Here's how the part is built. I have some questions about the finished solid (model axes, mm). A direction names the side the tool comes from. Give positions to 0.01 mm unless a question says otherwise; leave off trailing zeros. Loops run counter-clockwise (first coordinate to the right, second up) from the corner with the lowest first, then second, coordinate; pieces in that order, holes last.
Q1. Thinking about a two-plate mould opening in X: for faces 1 (the face through (39.6, 61.94, 12.68)), 2 (the face through (10, 50, 5)), 3 (the face through (20, 39, 25)), which applies, pulls with the +X half, pulls with the -X half, needs draft (parallel to the pull), parting line crosses it, or undercut?
Q2. I need wall thicknesses on probe 1 along Y at (x, z) = (10, 12); probe 2 along Y at (x, z) = (10, 16); probe 3 along Y at (x, z) = (10, 21.25). Which ranges of each line are inside material? Lowest first, please.
Q3. Suppose I cut it at B-B (x = 4). List the corners of the cut face in (y, z) for me.
Q4. I'm going to push flat-ended pins straight in: P1, Ø3, axis at x = 37.5, y = 28, coming from the +Z side; P2, Ø3, axis at x = 4, z = 16.5, coming from the -Y side; P3, Ø5, axis at x = 11.5, y = 31.5, coming from the +Z side. Where does each tip first touch, or does it pass through?
Q5. For faces 4 (the face through (30, 42, 20.1)), 5 (the face through (35, 36.14, 22)), 6 (the face through (29.25, 56, 17)), 7 (the face through (9.9, 28.8, 5)), which set-ups out of +Z, -Z, +X, -X, +Y, -Y let a thin tool reach every point of the face, with its end or its side?
Q6. Suppose I cut it at D-D (y = 41.65). List the corners of the cut face in (x, z) for me.
Q7. Suppose I cut it at A-A (y = 52.3). List the corners of the cut face in (x, z) for me, and give its area (4 significant figures).
Q8. Suppose I cut it at C-C (z = 15). List the corners of the cut face in (x, y) for me.
```python
from build123d import *

# Parameters (mm, degrees)
EXTRUDE_DEPTH     = 20
BOX003_W          = 15
BOX003_H          = 7.5
BOX003_DEPTH      = 6
CYLINDER003_R     = 2.1
CYLINDER003_DEPTH = 5
CYLINDER002_R     = 1.05
CYLINDER002_DEPTH = 7
BOX002_W          = 10
BOX002_H          = 13
BOX002_DEPTH      = 6
CYLINDER001_R     = 2
CYLINDER001_DEPTH = 5
CYLINDER_R        = 5
CYLINDER_DEPTH    = 20
BOX001_W          = 20.5
BOX001_H          = 20.5
BOX001_DEPTH      = 25
BOX004_W          = 7.5
BOX004_H          = 13
BOX004_DEPTH      = 6
BOX_W             = 40.5
BOX_H             = 62.8
BOX_DEPTH         = 25
FILLET_R          = 3


with BuildPart() as obj1:
    # Sketch → Extrude (new body)
    with BuildSketch(Plane.YZ):
        with BuildLine():
            ThreePointArc((-3.606243, 3.606246), (0, -5.1), (3.606243, 3.606246))
            Line((2.112489, 5.1), (3.606243, 3.606246))
            Line((-2.112489, 5.1), (2.112489, 5.1))
            Line((-3.606243, 3.606246), (-2.112489, 5.1))
        make_face()
    extrude(amount=EXTRUDE_DEPTH)


with BuildPart() as obj1_1:
    # Extrude placement: moved
    add(obj1.part.moved(Location((20.5, 41.65, 15))))


with BuildPart() as hueco_taladro4:
    # Box003 → Box003 (new body)
    with BuildSketch(Plane(origin=(0, 39, 14), x_dir=(1, 0, 0), z_dir=(0, 0, 1))):
        with Locations((7.5, 3.75)):
            Rectangle(BOX003_W, BOX003_H)
    extrude(amount=BOX003_DEPTH)


with BuildPart() as taladro4:
    # Cylinder003 → Cylinder003 (new body)
    with BuildSketch(Plane(origin=(10, 42.7, 20), x_dir=(1, 0, 0), z_dir=(0, 0, 1))):
        Circle(CYLINDER003_R)
    extrude(amount=CYLINDER003_DEPTH)


with BuildPart() as clone005:
    # Clone005 base: copy of taladro4
    add(taladro4.part)


with BuildPart() as clone005_1:
    # Clone005 placement: moved
    add(clone005.part.moved(Location((15.5, 13.1, 0))))


with BuildPart() as taladro_endstop:
    # Cylinder002 → Cylinder002 (new body)
    with BuildSketch(Plane(origin=(35.5, 26.14, 12), x_dir=(1, 0, 0), z_dir=(0, 0, 1))):
        Circle(CYLINDER002_R)
    extrude(amount=CYLINDER002_DEPTH)


with BuildPart() as clone004:
    # Clone004 base: copy of taladro_endstop
    add(taladro_endstop.part)


with BuildPart() as clone004_1:
    # Clone004 placement: moved
    add(clone004.part.moved(Location((0, 7, 0))))


with BuildPart() as hueco_endstop:
    # Box002 → Box002 (new body)
    with BuildSketch(Plane(origin=(30.5, 23.14, 19), x_dir=(1, 0, 0), z_dir=(0, 0, 1))):
        with Locations((5, 6.5)):
            Rectangle(BOX002_W, BOX002_H)
    extrude(amount=BOX002_DEPTH)


with BuildPart() as taladro5:
    # Cylinder001 → Cylinder001 (new body)
    with BuildSketch(Plane(origin=(30.5, 10, 0), x_dir=(1, 0, 0), z_dir=(0, 0, 1))):
        Circle(CYLINDER001_R)
    extrude(amount=CYLINDER001_DEPTH)


with BuildPart() as clone002:
    # Clone002 base: copy of taladro5
    add(taladro5.part)


with BuildPart() as clone002_1:
    # Clone002 placement: moved
    add(clone002.part.moved(Location((-20.5, 21, 0))))


with BuildPart() as clone003:
    # Clone003 base: copy of Clone002
    add(clone002_1.part)


with BuildPart() as clone003_1:
    # Clone003 placement: moved
    add(clone003.part.moved(Location((0, 21.3, 0))))


with BuildPart() as taladro10:
    # Cylinder → Cylinder (new body)
    with BuildSketch(Plane(origin=(30.5, 10, 5), x_dir=(1, 0, 0), z_dir=(0, 0, 1))):
        Circle(CYLINDER_R)
    extrude(amount=CYLINDER_DEPTH)


with BuildPart() as clone:
    # Clone base: copy of taladro10
    add(taladro10.part)


with BuildPart() as clone_1:
    # Clone placement: moved
    add(clone.part.moved(Location((-20.5, 21, 0))))


with BuildPart() as clone001:
    # Clone001 base: copy of Clone
    add(clone_1.part)


with BuildPart() as clone001_1:
    # Clone001 placement: moved
    add(clone001.part.moved(Location((0, 21.3, 0))))


with BuildPart() as obj2:
    # Box001 → Box001 (new body)
    with BuildSketch(Plane.XY):
        with Locations((10.25, 10.25)):
            Rectangle(BOX001_W, BOX001_H)
    extrude(amount=BOX001_DEPTH)


with BuildPart() as huecos:
    # Box004 → Box004 (new body)
    with BuildSketch(Plane(origin=(21.75, 49.8, 14), x_dir=(1, 0, 0), z_dir=(0, 0, 1))):
        with Locations((3.75, 6.5)):
            Rectangle(BOX004_W, BOX004_H)
    extrude(amount=BOX004_DEPTH)

    # Fusion: union hueco_taladro4, Clone005, taladro4, Clone004, taladro_endstop, hueco_endstop, Clone003, Clone002, taladro5, Clone001, Clone, taladro10, obj2
    add(hueco_taladro4.part)
    add(clone005_1.part)
    add(taladro4.part)
    add(clone004_1.part)
    add(taladro_endstop.part)
    add(hueco_endstop.part)
    add(clone003_1.part)
    add(clone002_1.part)
    add(taladro5.part)
    add(clone001_1.part)
    add(clone_1.part)
    add(taladro10.part)
    add(obj2.part)


with BuildPart() as obj3:
    # Box → Box (new body)
    with BuildSketch(Plane.XY):
        with Locations((20.25, 31.4)):
            Rectangle(BOX_W, BOX_H)
    extrude(amount=BOX_DEPTH)

    # Cut: cut huecos
    add(huecos.part, mode=Mode.SUBTRACT)

    # Cut001: cut obj1
    add(obj1_1.part, mode=Mode.SUBTRACT)

    # Fillet
    fillet_edges = [obj3.edges().sort_by_distance(p)[0] for p in [
        (0, 62.8, 12.5),
        (40.5, 62.8, 12.5),
        (40.5, 0, 12.5),
    ]]
    fillet(fillet_edges, radius=FILLET_R)


solid = obj3.part
```
Solutions:
1. face 1: pulls with the +X half
1. face 2: undercut
1. face 3: needs draft
2. probe 1: y = 20.5 to 26, 36 to 47.3, 57.3 to 62.8
2. probe 2: y = 20.5 to 26, 36 to 39, 46.5 to 47.3, 57.3 to 62.8
2. probe 3: y = 20.5 to 26, 36 to 40.6, 44.8 to 47.3, 57.3 to 62.8
3. outline: (20.5, 0) - (62.8, 0) - (62.8, 25) - (20.5, 25) - close; hole (39, 14) - (46.5, 14) - (46.5, 20) - (39, 20) - close
4. P1: stops at z = 19
4. P2: stops at y = 20.5
4. P3: stops at z = 5
5. face 4: +X
5. face 5: +Z, +X
5. face 6: +Y
5. face 7: +Z
6. outline: (0, 0) - (40.5, 0) - (40.5, 9.9) - (20.5, 9.9) - (20.5, 20.1) - (40.5, 20.1) - (40.5, 25) - (11.82, 25) - (11.82, 20) - (15, 20) - (15, 14) - (0, 14) - close; (0, 20) - (8.18, 20) - (8.18, 25) - (0, 25) - close
7. outline: (0, 0) - (8, 0) - (8, 5) - (5, 5) - (5, 25) - (0, 25) - close; (12, 0) - (40.5, 0) - (40.5, 25) - (15, 25) - (15, 5) - (12, 5) - close; hole (21.75, 14) - (29.25, 14) - (29.25, 20) - (21.75, 20) - close
7. area: 747.5 mm2
8. outline: (0, 20.5) - (20.5, 20.5) - (20.5, 0) - (37.5, 0) arc R3 ccw to (40.5, 3) - (40.5, 36.55) - (20.5, 36.55) - (20.5, 46.75) - (40.5, 46.75) - (40.5, 59.8) arc R3 ccw to (37.5, 62.8) - (29.25, 62.8) - (29.25, 49.8) - (21.75, 49.8) - (21.75, 62.8) - (3, 62.8) arc R3 ccw to (0, 59.8) - (0, 46.5) - (15, 46.5) - (15, 39) - (0, 39) - close; hole circle Ø10 at (10, 31); hole circle Ø10 at (10, 52.3); hole circle Ø10 at (30.5, 10); hole circle Ø2.1 at (35.5, 26.14); hole circle Ø2.1 at (35.5, 33.14)
